The model under review builds one solid part; all positions refer to its coordinate system, in mm. A direction names the side the tool comes from. Round coordinates to 2 decimals unless told otherwise and drop trailing zeros. Write each loop counter-clockwise with the first axis right and the second up, starting at its lowest first coordinate (ties: lowest second). Pieces come first, ordered by that corner, then holes.
Item 1: Add section D-D (z = -37). Give the boundary of the cut face in (x, y), plus the area to 3 significant figures.
Item 2: To check wall thickness, follow L1, parallel to Y at x = 59, z = -34; L2, parallel to Z at x = 22.5, y = -4.5; L3, parallel to Z at x = 24, y = 0.75. State the ranges of each line that lie inside material, in increasing order.
Item 3: Add section C-C (y = -6.25). Give the boundary of the cut face in (x, z), plus the area to 3 significant figures.
Item 4: Add section B-B (y = -2.25). Give the boundary of the cut face in (x, z), plus the area to 3 significant figures.
Item 5: Clearance check with flat-ended pins moving along their axes: pin 1 Ø2 at (x, z) = (57, -30) entering from -Y; pin 2 Ø1.6 at (x, y) = (36.5, 1.5) entering from -Z; pin 3 Ø0.6 at (y, z) = (-2.5, -65.5) entering from +X; pin 4 Ø1.5 at (x, y) = (58.5, 0.5) entering from +Z. State where each tip first meets the part, or that it passes through.
Item 6: Machinability: for faces 4 (the face through (7, 1, -64.7)), 5 (the face through (63, 1, -64.7)), 6 (the face through (19, -6, -64.7)), 7 (the face through (19, -1, -66)), which of the approach directions +Z, -Z, +X, -X, +Y, -Y give a long, thin tool a straight path to every point of the face, cutting with its end or side? Answer none if there is none.
Item 7: Draft analysis for pull direction Y (two halves, no side actions). For faces 1 (the face through (52, -6, -64.7)), 2 (the face through (52, -8, -66)), 3 (the face through (54, -3, -66)), state which applies: +Y half, -Y half, draft (parallel to the pull), parting line (faces both ways), or undercut.
Item 8: Add section A-A (x = 52). Give the boundary of the cut face in (y, z), plus the area to 3 significant figures.
```python
from build123d import *

# Parameters (mm, degrees)
SKETCH1_W           = 70
SKETCH1_H           = 64.7
BOSS_EXTRUDE1_DEPTH = 2
SKETCH2_W           = 10
SKETCH2_H           = 10
SKETCH2_W_2         = 5
SKETCH2_H_2         = 4
BOSS_EXTRUDE2_DEPTH = 2
FILLET2_R           = 0.2


with BuildPart() as part:
    # Sketch1 → Boss-Extrude1 (new body)
    with BuildSketch(Plane(origin=(0, 0, 0), x_dir=(1, 0, 0), z_dir=(0, 1, 0))):
        with Locations((35, 32.35)):
            Rectangle(SKETCH1_W, SKETCH1_H)
    extrude(amount=BOSS_EXTRUDE1_DEPTH)

    # Sketch2 → Boss-Extrude2 (add)
    # profile 1 of 2: a face of its own
    with BuildSketch(Plane(origin=(0, 0, -64.7), x_dir=(-1, 0, 0), z_dir=(0, 0, -1))):
        with Locations((-51.5, -3)):
            Rectangle(SKETCH2_W, SKETCH2_H)
        with Locations((-51.5, -3)):
            Rectangle(SKETCH2_W_2, SKETCH2_H_2, mode=Mode.SUBTRACT)
    # profile 2 of 2: a face of its own
    with BuildSketch(Plane(origin=(0, 0, -64.7), x_dir=(-1, 0, 0), z_dir=(0, 0, -1))):
        with Locations((-18.5, -3)):
            Rectangle(SKETCH2_W, SKETCH2_H)
        with Locations((-18.5, -3)):
            Rectangle(SKETCH2_W_2, SKETCH2_H_2, mode=Mode.SUBTRACT)
    extrude(amount=BOSS_EXTRUDE2_DEPTH)

    # Fillet2
    # the kernel refuses this fillet: 0.2 mm, written as the material it adds along each edge
    with BuildSketch(Plane(origin=(13.5, 0, -64.7), x_dir=(-1, 0, 0), z_dir=(0, 1, 0)), Plane(origin=(23.5, 2, -64.7), x_dir=(1, 0, 0), z_dir=(0, -1, 0)), Plane(origin=(21, -5, -64.7), x_dir=(0, 1, 0), z_dir=(0, 0, -1)), Plane(origin=(16, -5, -64.7), x_dir=(1, 0, 0), z_dir=(0, 0, -1)), Plane(origin=(49, -5, -64.7), x_dir=(1, 0, 0), z_dir=(0, 0, -1)), Plane(origin=(49, -1, -64.7), x_dir=(0, -1, 0), z_dir=(0, 0, -1))) as fillet2_piece_1:
        with BuildLine():
            CenterArc((FILLET2_R, -FILLET2_R), FILLET2_R, 90, 90)
            Line((0, -FILLET2_R), (0, 0))
            Line((0, 0), (FILLET2_R, 0))
        make_face()
    extrude(amount=2)
    with BuildSketch(Plane(origin=(56.5, 0, -64.7), x_dir=(1, 0, 0), z_dir=(0, 1, 0)), Plane(origin=(46.5, 2, -64.7), x_dir=(-1, 0, 0), z_dir=(0, -1, 0)), Plane(origin=(21, -1, -64.7), x_dir=(0, -1, 0), z_dir=(0, 0, -1)), Plane(origin=(16, -1, -64.7), x_dir=(1, 0, 0), z_dir=(0, 0, -1)), Plane(origin=(54, -1, -64.7), x_dir=(0, -1, 0), z_dir=(0, 0, -1)), Plane(origin=(54, -5, -64.7), x_dir=(-1, 0, 0), z_dir=(0, 0, -1))) as fillet2_piece_2:
        with BuildLine():
            CenterArc((FILLET2_R, FILLET2_R), FILLET2_R, 180, 90)
            Line((0, FILLET2_R), (0, 0))
            Line((0, 0), (FILLET2_R, 0))
        make_face()
    extrude(amount=2)
    # the kernel refuses this fillet: 0.2 mm, written as the material it takes off along each edge
    with BuildSketch(Plane(origin=(13.5, 2, -64.9), x_dir=(1, 0, 0), z_dir=(0, 0, -1)), Plane(origin=(46.5, 2, -64.9), x_dir=(1, 0, 0), z_dir=(0, 0, -1))) as fillet2_2_piece_1:
        with BuildLine():
            CenterArc((FILLET2_R, FILLET2_R), FILLET2_R, 180, 90)
            Line((0, FILLET2_R), (0, 0))
            Line((0, 0), (FILLET2_R, 0))
        make_face()
    extrude(amount=2.3, mode=Mode.SUBTRACT)
    with BuildSketch(Plane(origin=(13.5, -8, -64.2), x_dir=(0, 1, 0), z_dir=(0, 0, -1)), Plane(origin=(46.5, -8, -64.2), x_dir=(0, 1, 0), z_dir=(0, 0, -1))) as fillet2_2_piece_2:
        with BuildLine():
            CenterArc((FILLET2_R, FILLET2_R), FILLET2_R, 180, 90)
            Line((0, FILLET2_R), (0, 0))
            Line((0, 0), (FILLET2_R, 0))
        make_face()
    extrude(amount=3, mode=Mode.SUBTRACT)
    with BuildSketch(Plane(origin=(23.5, -8, -64.2), x_dir=(0, 1, 0), z_dir=(0, 0, -1)), Plane(origin=(56.5, -8, -64.2), x_dir=(0, 1, 0), z_dir=(0, 0, -1))) as fillet2_2_piece_3:
        with BuildLine():
            CenterArc((FILLET2_R, -FILLET2_R), FILLET2_R, 90, 90)
            Line((0, -FILLET2_R), (0, 0))
            Line((0, 0), (FILLET2_R, 0))
        make_face()
    extrude(amount=3, mode=Mode.SUBTRACT)
    with BuildSketch(Plane(origin=(23.5, 2, -64.9), x_dir=(-1, 0, 0), z_dir=(0, 0, -1)), Plane(origin=(56.5, 2, -64.9), x_dir=(-1, 0, 0), z_dir=(0, 0, -1))) as fillet2_2_piece_4:
        with BuildLine():
            CenterArc((FILLET2_R, -FILLET2_R), FILLET2_R, 90, 90)
            Line((0, -FILLET2_R), (0, 0))
            Line((0, 0), (FILLET2_R, 0))
        make_face()
    extrude(amount=2.3, mode=Mode.SUBTRACT)
    with BuildSketch(Plane(origin=(46.3, 2, -64.9), x_dir=(-0.5976672776327815, 0, -0.8017442392976825), z_dir=(0.8017442392976825, 0, -0.5976672776327815))) as fillet2_2_piece_5:
        with BuildLine():
            CenterArc((0.2 + FILLET2_R, -FILLET2_R), FILLET2_R, 90, 90)
            Line((0.2, -FILLET2_R), (0.2, 0))
            Line((0.2, 0), (0.2 + FILLET2_R, 0))
        make_face()
    revolve(axis=Axis((46.3, 2, -64.9), (0, 1, 0)), revolution_arc=233.296989237, mode=Mode.SUBTRACT)
    with BuildSketch(Plane(origin=(56.7, 2, -64.9), x_dir=(0.5976672776327815, 0, -0.8017442392976825), z_dir=(-0.8017442392976825, 0, -0.5976672776327815))) as fillet2_2_piece_6:
        with BuildLine():
            CenterArc((0.2 + FILLET2_R, FILLET2_R), FILLET2_R, 180, 90)
            Line((0.2, FILLET2_R), (0.2, 0))
            Line((0.2, 0), (0.2 + FILLET2_R, 0))
        make_face()
    revolve(axis=Axis((56.7, 2, -64.9), (0, -1, 0)), revolution_arc=233.296989237, mode=Mode.SUBTRACT)
    with BuildSketch(Plane(origin=(23.7, 2, -64.9), x_dir=(0.5976672776328044, 0, -0.8017442392976655), z_dir=(-0.8017442392976655, 0, -0.5976672776328044))) as fillet2_2_piece_7:
        with BuildLine():
            CenterArc((0.2 + FILLET2_R, FILLET2_R), FILLET2_R, 180, 90)
            Line((0.2, FILLET2_R), (0.2, 0))
            Line((0.2, 0), (0.2 + FILLET2_R, 0))
        make_face()
    revolve(axis=Axis((23.7, 2, -64.9), (0, -1, 0)), revolution_arc=233.296989237, mode=Mode.SUBTRACT)
    with BuildSketch(Plane(origin=(13.3, 2, -64.9), x_dir=(-0.5976672776327986, 0, -0.8017442392976697), z_dir=(0.8017442392976697, 0, -0.5976672776327986))) as fillet2_2_piece_8:
        with BuildLine():
            CenterArc((0.2 + FILLET2_R, -FILLET2_R), FILLET2_R, 90, 90)
            Line((0.2, -FILLET2_R), (0.2, 0))
            Line((0.2, 0), (0.2 + FILLET2_R, 0))
        make_face()
    revolve(axis=Axis((13.3, 2, -64.9), (0, 1, 0)), revolution_arc=233.296989237, mode=Mode.SUBTRACT)


solid = part.part
```
Numbers:
1. outline: (0, 0) - (70, 0) - (70, 2) - (0, 2) - close
1. area: 140 mm2
2. L1: y = 0 to 2
2. L2: z = -66.7 to -64.7
2. L3: z = -64.7 to 0
3. outline: (13.5, -66.7) - (23.5, -66.7) - (23.5, -64.7) - (13.5, -64.7) - close; (46.5, -66.7) - (56.5, -66.7) - (56.5, -64.7) - (46.5, -64.7) - close
3. area: 40.0 mm2
4. outline: (13.5, -66.7) - (16, -66.7) - (16, -64.7) - (13.5, -64.7) - close; (21, -66.7) - (23.5, -66.7) - (23.5, -64.7) - (21, -64.7) - close; (46.5, -66.7) - (49, -66.7) - (49, -64.7) - (46.5, -64.7) - close; (54, -66.7) - (56.5, -66.7) - (56.5, -64.7) - (54, -64.7) - close
4. area: 20.0 mm2
5. pin 1: stops at y = 0
5. pin 2: stops at z = -64.7
5. pin 3: stops at x = 56.5
5. pin 4: stops at z = 0
6. face 4: -Z, -X, +Y, -Y
6. face 5: -Z, +X, +Y, -Y
6. face 6: +Z, +X, -X, -Y
6. face 7: +Z, -Z
7. face 1: draft
7. face 2: -Y half
7. face 3: undercut
8. outline: (-8, -66.7) - (-5, -66.7) - (-5, -64.7) - (-8, -64.7) - close; (-1, -66.7) - (2, -66.7) - (2, 0) - (0, 0) - (0, -64.7) - (-1, -64.7) - close
8. area: 141 mm2
